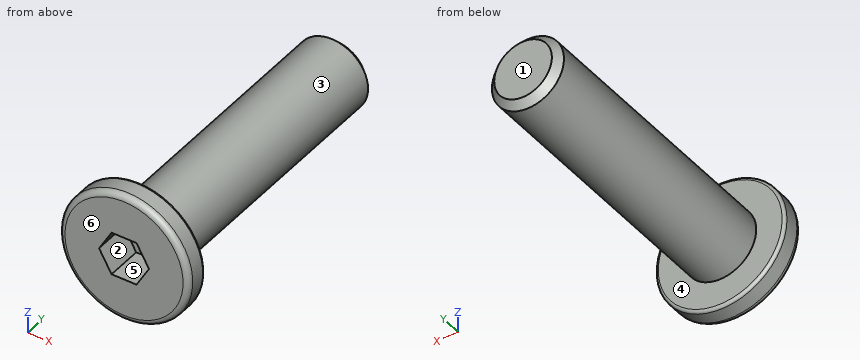
Autodesk Inventor part; units mm, degrees
ref_plane "YZ Plane" through (0, 0, 0) normal (1, 0, 0) x (0, 1, 0)
ref_plane "XZ Plane" through (0, 0, 0) normal (0, 1, 0) x (-1, 0, 0)
ref_plane "XY Plane" through (0, 0, 0) normal (0, 0, 1) x (1, 0, 0)
sketch "Boceto1" plane through (0, 0, 0) normal (0, 1, 0) x (-1, 0, 0)
  circle A0 centre (0, 0) radius 4.5
  dimension "d0" = 9
extrude "Extrusión1" add sketch "Boceto1" along normal blind 1.6
sketch "Boceto2" plane through (0, 1.6, 0) normal (0, 1, 0) x (1, 0, 0)
  circle A0 centre (0, 0) radius 2.5
  dimension "d3" = 5
extrude "Extrusión2" add sketch "Boceto2" along normal blind 20
fillet "Empalme1" radius 0.4 1 edges at (4.5, 0, 0)
fillet "Empalme2" radius 0.2 1 edges at (4.5, 1.6, 0)
sketch "Boceto3" plane through (0, 0, 0) normal (0, -1, 0) x (1, 0, 0)
  line L0 (-1.7321, 0) -> (-0.866, 1.5)
  line L1 (-0.866, 1.5) -> (0.866, 1.5)
  line L2 (0.866, 1.5) -> (1.7321, 0)
  line L3 (1.7321, 0) -> (0.866, -1.5)
  line L4 (0.866, -1.5) -> (-0.866, -1.5)
  line L5 (-0.866, -1.5) -> (-1.7321, 0)
  point P0 (0, 0)
  point P1 (0, 0)
  dimension "d8" = 3
extrude "Extrusión3" cut sketch "Boceto3" against normal blind 2.5
chamfer "Chaflán1" distance 0.5 angle 45 1 edges at (-2.5, 21.6, 0)
thread "Rosca2"
properties part number "Perno M5x8 cabeza plana" material "Hierro, gris"
Here's how the part is built. I have some questions about the finished solid (model axes, mm). Face numbers are marked on the shaded views. A direction names the side the tool comes from. Give positions to 0.01 mm unless a question says otherwise; leave off trailing zeros. Loops run counter-clockwise (first coordinate to the right, second up) from the corner with the lowest first, then second, coordinate; pieces in that order, holes last. Notation, with made-up numbers: M 66,22 L 78,22 A31 cw 78,54 Z; hole C 52,39.25 d11. An arc over 180 degrees is marked long. Put each result on its own line as item: value. Start each with the question number.
(1) Will these pins go through, and if not, where does the flat tip stop? pin 1 Ø2 at (y, z) = (11.5, 3) entering from +X; pin 2 Ø1.5 at (x, y) = (-1, 7.5) entering from +Z; pin 3 Ø4 at (y, z) = (8.5, 2) entering from +X.
(2) If we mould it in two halves opening along X, with no side actions, what happens to the marked faces 1, 2 and 3? For each: +X half, -X half, draft (parallel to the pull), parting line (faces both ways), or undercut.
(3) For the marked faces 4, 5 and 6, which set-ups out of +Z, -Z, +X, -X, +Y, -Y let a thin tool reach every point of the face, with its end or its side?
(4) I want a section at B-B on y = 3. Please give me the cut outline in (x, z), then the cut area to 3 significant figures.
(5) I need wall thicknesses on line 1 along Z through (x, y) = (-1.5, 4.75); line 2 along Y through (x, z) = (-3.5, 1); line 3 along Y through (x, z) = (0.25, -0.5). Which ranges of each line are inside material? Lowest first, please. Write a range as [from, to].
(6) I want a section at A-A on x = 0. Please give me the cut outline in (y, z), then the cut area to 3 significant figures.
Answer block:
1. pin 1: x = 1.5
1. pin 2: z = 2.49
1. pin 3: x = 2.5
2. face 1: draft
2. face 2: undercut
2. face 3: parting line
3. face 4: +Y
3. face 5: -Y
3. face 6: +Z, -Z, +X, -X, -Y
4. outline: C 0,0 d5
4. area: 19.6 mm^2
5. line 1: [-2, 2]
5. line 2: [0, 1.6]
5. line 3: [2.5, 21.6]
6. outline: M 0,-4.1 A0.4 ccw 0.4,-4.5 L 1.4,-4.5 A0.2 ccw 1.6,-4.3 L 1.6,-2.5 L 21.1,-2.5 L 21.6,-2 L 21.6,2 L 21.1,2.5 L 1.6,2.5 L 1.6,4.3 A0.2 ccw 1.4,4.5 L 0.4,4.5 A0.4 ccw 0,4.1 L 0,1.5 L 2.5,1.5 L 2.5,-1.5 L 0,-1.5 Z
6. area: 107 mm^2
